Check sheet for the modelled part. Datum: model origin and axes. Units: mm. A direction names the side the tool comes from. Give positions to 0.01 mm unless a question says otherwise; leave off trailing zeros. Write each loop counter-clockwise with the first axis right and the second up, starting at its lowest first coordinate (ties: lowest second). Pieces come first, ordered by that corner, then holes. Notation, with made-up numbers: (-12.5, 34.25) -> (25.5, 34.25) arc R36 ccw to (25.5, 69.25) -> close; hole circle Ø7 at (52, 82). An arc over 180 degrees is marked (long way). Answer as a JSON object with one key per item and string values.
from build123d import *

# Parameters (mm, degrees)
F0_W     = 12.7
F0_H     = 100
F0_R     = 2.5
F1_DEPTH = 12.7
F3_D     = 4.2
F4_W     = 3.175
F4_H     = 21
F5_DEPTH = 12.701
F6_DEPTH = 1


with BuildPart() as f1:
    # F0 (on Front) → F1 (new body)
    with BuildSketch(Plane.XZ):
        Rectangle(F0_W, F0_H)
        with Locations((0, -42.5)):
            Circle(F0_R, mode=Mode.SUBTRACT)
        with Locations((0, -22.5)):
            Circle(F0_R, mode=Mode.SUBTRACT)
    extrude(amount=F1_DEPTH)

    # F3 (through all)
    with Locations(Plane.XZ.offset(12.7)):
        with Locations((0, 45), (0, 34)):
            Hole(F3_D / 2)

    # F4 (on face) → F5 (cut, through all)
    with BuildSketch(Plane(origin=(-6.35, 0, 0), x_dir=(0, -1, 0), z_dir=(-1, 0, 0))):
        with Locations((1.5875, 39.5)):
            Rectangle(F4_W, F4_H)
        with Locations((11.1125, 39.5)):
            Rectangle(F4_W, F4_H)
    extrude(amount=-F5_DEPTH, mode=Mode.SUBTRACT)

    # F6 (add): a face of the model
    f6_faces = [f1.faces().sort_by_distance(p)[0] for p in [
        (-6.35, -6.35, -4.6340782123),
    ]]
    extrude(f6_faces, amount=F6_DEPTH)


solid = f1.part
1. Sectioned sample at D-D, the plane x = 4.5. Enter the section's corners in (y, z) (3 decimals).
Determined:
{"outline": "(-12.7, -50) -> (0, -50) -> (0, 29) -> (-3.175, 29) -> (-3.175, 50) -> (-9.525, 50) -> (-9.525, 29) -> (-12.7, 29) -> close"}
2. Go/stop test with flat-tipped pins: P1, Ø1.5, axis at x = 2, y = -10.5, coming from the +Z side; P2, Ø4, axis at x = -2, z = 38.5, coming from the +Y side (3 decimals); P3, Ø5, axis at x = 0, z = 34, coming from the -Y side (3 decimals). Record where each tip stops, or that it passes through.
Determined:
{"P1": "z = 29", "P2": "y = -3.175", "P3": "y = -9.525"}
3. Sectioned sample at C-C, the plane z = 34. Enter the section's corners in (x, y) (3 decimals), plus the area to 3 significant figures.
Determined:
{"outline": "(-7.35, -9.525) -> (-2.1, -9.525) -> (-2.1, -3.175) -> (-7.35, -3.175) -> close; (2.1, -9.525) -> (6.35, -9.525) -> (6.35, -3.175) -> (2.1, -3.175) -> close", "area": "60.3 mm^2"}
4. Mould release check, pull along X, two halves, no side actions. Record for faces 1 (the face through (0, -11, 29)), 2 (the face through (6.35, -6, -1)), 3 (the face through (-0.54, -6.26, -44.94)): released by +X, released by -X, zero draft, split by the parting line, or undercut.
Determined:
{"face 1": "zero draft", "face 2": "released by +X", "face 3": "undercut"}
5. Sectioned sample at A-A, the plane z = -22.5. Enter the section's corners in (x, y).
Determined:
{"outline": "(-7.35, -12.7) -> (-2.5, -12.7) -> (-2.5, 0) -> (-7.35, 0) -> close; (2.5, -12.7) -> (6.35, -12.7) -> (6.35, 0) -> (2.5, 0) -> close"}
6. Scan lines: L1, parallel to Z at x = 0, y = -8; L2, parallel to Z at x = 0, y = -2.5; L3, parallel to Y at x = -0.75, z = 38 (3 decimals). Record each from-to range of solid material in increasing order. Write a range as [from, to].
Determined:
{"L1": "[-50, -45], [-40, -25], [-20, 31.9], [36.1, 42.9], [47.1, 50]", "L2": "[-50, -45], [-40, -25], [-20, 29]", "L3": "[-9.525, -3.175]"}
7. Access from +Z, -Z, +X, -X, +Y, -Y to the whole of each face (thin tool, end or side, straight path). Record for faces 4 (the face through (0, -2, 29)), 5 (the face through (0, -9.525, 39)), 6 (the face through (0, -6, -50)).
Determined:
{"face 4": "+Z, +X, -X, +Y", "face 5": "+Z, +X, -X, -Y", "face 6": "-Z, +X, -X, +Y, -Y"}
8. Sectioned sample at B-B, the plane x = 0. Enter the section's corners in (y, z) (3 decimals), plus the area to 3 significant figures.
Determined:
{"outline": "(-12.7, -50) -> (0, -50) -> (0, -45) -> (-12.7, -45) -> close; (-12.7, -40) -> (0, -40) -> (0, -25) -> (-12.7, -25) -> close; (-12.7, -20) -> (0, -20) -> (0, 29) -> (-3.175, 29) -> (-3.175, 31.9) -> (-9.525, 31.9) -> (-9.525, 29) -> (-12.7, 29) -> close; (-9.525, 36.1) -> (-3.175, 36.1) -> (-3.175, 42.9) -> (-9.525, 42.9) -> close; (-9.525, 47.1) -> (-3.175, 47.1) -> (-3.175, 50) -> (-9.525, 50) -> close", "area": "956 mm^2"}
